Model file for the job. Use its own axes, mm. A direction names the side the tool comes from. Coordinates: 2 decimals unless noted, no trailing zeros. Write each loop counter-clockwise with the first axis right and the second up, starting at its lowest first coordinate (ties: lowest second). Pieces come first, ordered by that corner, then holes.
Q1. Band-saw the part on A-A, the plane x = 0. Write the cut outline in (y, z).
Q2. Band-saw the part on D-D, the plane y = -4. Write the cut outline in (x, z), plus the area to 3 significant figures.
Q3. Band-saw the part on B-B, the plane y = 22. Write the cut outline in (x, z), plus the area to 3 significant figures.
Q4. Pull direction X, two halves, no side cores. Call faces 4 (the flat face through (0, 20, 10)), 5 (the flat face through (0, -12.5, 0)), 6 (the cylindrical face through (8.86, -6.16, -28.14)): released by +X, released by -X, zero draft, split by the parting line, or undercut.
Q5. Pin check, flat tips, straight feed: P1, Ø1.8, axis at x = 29.44, z = -17, coming from the -Y side; P2, Ø2.5, axis at x = -29.44, z = 17, coming from the +Y side; P3, Ø1.5, axis at x = -14, y = 14.5, coming from the -Z side. Stop position of each tip, or through.
Q6. Drill centre lines: probe 1 along X at (y, z) = (0.9, -17); probe 2 along Z at (x, y) = (-30, 1); probe 3 along X at (y, z) = (1, -34). Where is each one in solid material? Low to high.
Q7. Band-saw the part on C-C, the plane z = 0.5. Write the cut outline in (x, y).
Q8. Which spindle directions (+Z, -Z, +X, -X, +Y, -Y) get a long thin tool onto all of the face, cutting with end or side? Do faces 1 (the cylindrical face through (-27.96, 1.48, 17.2)), 2 (the cylindrical face through (-23.122, 12.078, -30.156)), 3 (the flat face through (1, 24.5, 16)). Say none if no direction does.
from build123d import *

# Parameters (mm, degrees)
SKETCH1_R           = 38
BOSS_EXTRUDE1_DEPTH = 24.5
SKETCH2_R           = 14
BOSS_EXTRUDE2_DEPTH = 0.5
SKETCH3_R           = 29.5
BOSS_EXTRUDE3_DEPTH = 12.5
SKETCH4_R           = 1.5
CUT_EXTRUDE1_DEPTH  = 5
SKETCH8_R           = 1.5
CUT_EXTRUDE3_DEPTH  = 3


with BuildPart() as part:
    # Sketch1 → Boss-Extrude1 (new body)
    with BuildSketch(Plane(origin=(0, 0, 0), x_dir=(1, 0, 0), z_dir=(0, 1, 0))):
        with Locations(Location((0, 0, 0), (0, 0, 270))):
            Circle(SKETCH1_R)
    extrude(amount=BOSS_EXTRUDE1_DEPTH)

    # Sketch2 → Boss-Extrude2 (add)
    with BuildSketch(Plane(origin=(0, 24.5, 0), x_dir=(1, 0, 0), z_dir=(0, 1, 0))):
        with Locations(Location((0, 0, 0), (0, 0, 270))):
            Circle(SKETCH2_R)
    extrude(amount=BOSS_EXTRUDE2_DEPTH)

    # Sketch3 → Boss-Extrude3 (add)
    with BuildSketch(Plane.XZ):
        with Locations(Location((0, 0, 0), (0, 0, 270))):
            Circle(SKETCH3_R)
    extrude(amount=BOSS_EXTRUDE3_DEPTH)

    # Sketch4 → Cut-Extrude1 (cut)
    with BuildSketch(Plane(origin=(0, 25, 0), x_dir=(1, 0, 0), z_dir=(0, 1, 0))):
        with Locations(Location((0, 10, 0), (0, 0, 270))):
            Circle(SKETCH4_R)
        with Locations(Location((8.660254038, 5, 0), (0, 0, 270))):
            Circle(SKETCH4_R)
        with Locations(Location((8.660254038, -5, 0), (0, 0, 270))):
            Circle(SKETCH4_R)
        with Locations(Location((0, -10, 0), (0, 0, 270))):
            Circle(SKETCH4_R)
        with Locations(Location((-8.660254038, -5, 0), (0, 0, 270))):
            Circle(SKETCH4_R)
        with Locations(Location((-8.660254038, 5, 0), (0, 0, 270))):
            Circle(SKETCH4_R)
    extrude(amount=-CUT_EXTRUDE1_DEPTH, mode=Mode.SUBTRACT)

    # Sketch8 → Cut-Extrude3 (cut)
    with BuildSketch(Plane.XZ):
        with Locations(Location((0, 34, 0), (0, 0, 270))):
            Circle(SKETCH8_R)
        with Locations(Location((29.444863729, 17, 0), (0, 0, 270))):
            Circle(SKETCH8_R)
        with Locations(Location((29.444863729, -17, 0), (0, 0, 270))):
            Circle(SKETCH8_R)
        with Locations(Location((0, -34, 0), (0, 0, 270))):
            Circle(SKETCH8_R)
        with Locations(Location((-29.444863729, -17, 0), (0, 0, 270))):
            Circle(SKETCH8_R)
        with Locations(Location((-29.444863729, 17, 0), (0, 0, 270))):
            Circle(SKETCH8_R)
    extrude(amount=-CUT_EXTRUDE3_DEPTH, mode=Mode.SUBTRACT)


solid = part.part
Answer sheet:
1. outline: (-12.5, -29.5) - (0, -29.5) - (0, -32.5) - (3, -32.5) - (3, -35.5) - (0, -35.5) - (0, -38) - (24.5, -38) - (24.5, -14) - (25, -14) - (25, -11.5) - (20, -11.5) - (20, -8.5) - (25, -8.5) - (25, 8.5) - (20, 8.5) - (20, 11.5) - (25, 11.5) - (25, 14) - (24.5, 14) - (24.5, 38) - (0, 38) - (0, 35.5) - (3, 35.5) - (3, 32.5) - (0, 32.5) - (0, 29.5) - (-12.5, 29.5) - close
2. outline: circle Ø59 at (0, 0)
2. area: 2,730 mm2
3. outline: circle Ø76 at (0, 0); hole circle Ø3 at (-8.66, -5); hole circle Ø3 at (-8.66, 5); hole circle Ø3 at (0, -10); hole circle Ø3 at (0, 10); hole circle Ø3 at (8.66, -5); hole circle Ø3 at (8.66, 5)
3. area: 4,490 mm2
4. face 4: undercut
4. face 5: zero draft
4. face 6: split by the parting line
5. P1: stops at y = 3
5. P2: stops at y = 24.5
5. P3: stops at z = -35.62
6. probe 1: x = -33.99 to -30.94, -27.94 to 27.94, 30.94 to 33.99
6. probe 2: z = -23.32 to -18.39, -15.61 to 15.61, 18.39 to 23.32
6. probe 3: x = -16.97 to -1.5, 1.5 to 16.97
7. outline: (-38, 0) - (-29.5, 0) - (-29.5, -12.5) - (29.5, -12.5) - (29.5, 0) - (38, 0) - (38, 24.5) - (13.99, 24.5) - (13.99, 25) - (-13.99, 25) - (-13.99, 24.5) - (-38, 24.5) - close
8. face 1: -Y
8. face 2: +Y, -Y
8. face 3: +Y
